For this review, take the finished solid that the model builds, in its own axes (mm). Coordinates: 2 decimals unless noted, no trailing zeros. Loops run counter-clockwise (first coordinate to the right, second up) from the corner with the lowest first, then second, coordinate; pieces in that order, holes last. Notation, with made-up numbers: (12.5, 21.25) -> (59.5, 21.25) arc R18 cw to (59.5, 25.25) -> close; hole circle Ø4 at (21, -37). An arc over 180 degrees is marked (long way). Answer in a Markdown table with one row per item.
from build123d import *

# Parameters (mm, degrees)
SKETCH1_W           = 457.2
SKETCH1_H           = 609.6
SKETCH1_W_2         = 250
SKETCH1_H_2         = 449.2
BOSS_EXTRUDE1_DEPTH = 1.5875


with BuildPart() as part:
    # Sketch1 → Boss-Extrude1 (new body, symmetric)
    with BuildSketch(Plane(origin=(0, 0, 0), x_dir=(1, 0, 0), z_dir=(0, 1, 0))):
        Rectangle(SKETCH1_W, SKETCH1_H)
        with Locations((0, -29.4)):
            Rectangle(SKETCH1_W_2, SKETCH1_H_2, mode=Mode.SUBTRACT)
    extrude(amount=BOSS_EXTRUDE1_DEPTH, both=True)


solid = part.part
Item 1: Take a section at B-B, the plane z = 93. State the section outline as (x, y) points, and give its area (3 significant figures).
Worked answers:
| item | result |
|---|---|
| outline | (-228.6, -1.59) -> (-125, -1.59) -> (-125, 1.59) -> (-228.6, 1.59) -> close; (125, -1.59) -> (228.6, -1.59) -> (228.6, 1.59) -> (125, 1.59) -> close |
| area | 658 mm² |
Item 2: Take a section at C-C, the plane y = 0.5. State the section outline as (x, z) points.
Worked answers:
| item | result |
|---|---|
| outline | (-228.6, -304.8) -> (228.6, -304.8) -> (228.6, 304.8) -> (-228.6, 304.8) -> close; hole (-125, -195.2) -> (125, -195.2) -> (125, 254) -> (-125, 254) -> close |
Item 3: Take a section at A-A, the plane x = 109. State the section outline as (y, z) points.
Worked answers:
| item | result |
|---|---|
| outline | (-1.59, -304.8) -> (1.59, -304.8) -> (1.59, -195.2) -> (-1.59, -195.2) -> close; (-1.59, 254) -> (1.59, 254) -> (1.59, 304.8) -> (-1.59, 304.8) -> close |
Item 4: For L1, parallel to Z at x = -92, y = -1.05; L2, parallel to X at y = -1, z = 198, list the stretches that pass through material, from the lowest coordinate up.
Worked answers:
| item | result |
|---|---|
| L1 | -304.8 to -195.2, 254 to 304.8 |
| L2 | -228.6 to -125, 125 to 228.6 |
